from build123d import *

# Parameters (mm, degrees)
SKETCH1_R           = 15
SKETCH1_R_2         = 10
BOSS_EXTRUDE1_DEPTH = 65
SKETCH2_R           = 25
SKETCH2_R_2         = 10
SKETCH2_R_3         = 2.25
BOSS_EXTRUDE2_DEPTH = 4
SKETCH4_R           = 1.4
CUT_EXTRUDE1_DEPTH  = 20
CHAMFER1_SIZE       = 1
CHAMFER2_SIZE       = 0.5
FILLET1_R           = 0.5


with BuildPart() as part:
    # Sketch1 → Boss-Extrude1 (new body)
    with BuildSketch(Plane(origin=(0, 0, 0), x_dir=(1, 0, 0), z_dir=(0, 1, 0))):
        with Locations(Location((0, 0, 0), (0, 0, 270))):
            Circle(SKETCH1_R)
        with Locations(Location((0, 0, 0), (0, 0, 270))):
            Circle(SKETCH1_R_2, mode=Mode.SUBTRACT)
    extrude(amount=BOSS_EXTRUDE1_DEPTH)

    # Sketch2 → Boss-Extrude2 (add)
    with BuildSketch(Plane(origin=(0, 65, 0), x_dir=(1, 0, 0), z_dir=(0, 1, 0))):
        with Locations(Location((0, 0, 0), (0, 0, 270))):
            Circle(SKETCH2_R)
        with Locations(Location((0, 0, 0), (0, 0, 270))):
            Circle(SKETCH2_R_2, mode=Mode.SUBTRACT)
        with Locations(Location((20, 0, 0), (0, 0, 270))):
            Circle(SKETCH2_R_3, mode=Mode.SUBTRACT)
        with Locations(Location((0, -20, 0), (0, 0, 270))):
            Circle(SKETCH2_R_3, mode=Mode.SUBTRACT)
        with Locations(Location((-20, 0, 0), (0, 0, 270))):
            Circle(SKETCH2_R_3, mode=Mode.SUBTRACT)
        with Locations(Location((0, 20, 0), (0, 0, 270))):
            Circle(SKETCH2_R_3, mode=Mode.SUBTRACT)
    extrude(amount=BOSS_EXTRUDE2_DEPTH)

    # Sketch4 → Cut-Extrude1 (cut)
    with BuildSketch(Plane.XZ):
        with Locations(Location((12.5, 0, 0), (0, 0, 270))):
            Circle(SKETCH4_R)
        with Locations(Location((0, -12.5, 0), (0, 0, 270))):
            Circle(SKETCH4_R)
        with Locations(Location((-12.5, 0, 0), (0, 0, 270))):
            Circle(SKETCH4_R)
        with Locations(Location((0, 12.5, 0), (0, 0, 270))):
            Circle(SKETCH4_R)
    extrude(amount=-CUT_EXTRUDE1_DEPTH, mode=Mode.SUBTRACT)

    # Chamfer1
    chamfer1_edges = [part.edges().sort_by_distance(p)[0] for p in [
        (0, 0, -15),
    ]]
    chamfer(chamfer1_edges, length=CHAMFER1_SIZE)

    # Chamfer2
    chamfer2_edges = [part.edges().sort_by_distance(p)[0] for p in [
        (0, 65, -25),
    ]]
    chamfer(chamfer2_edges, length=CHAMFER2_SIZE)

    # Fillet1
    fillet1_edges = [part.edges().sort_by_distance(p)[0] for p in [
        (0, 65, -15),
    ]]
    fillet(fillet1_edges, radius=FILLET1_R)


solid = part.part
Can you work these out from the model? Positions are in its coordinate system, mm. A direction names the side the tool comes from. Coordinates: 2 decimals unless noted, no trailing zeros. Write each loop counter-clockwise with the first axis right and the second up, starting at its lowest first coordinate (ties: lowest second). Pieces come first, ordered by that corner, then holes.
Q1. Please list where these lines run through material, in increasing order: L1, parallel to X at y = 66, z = 20; L2, parallel to X at y = 46, z = 0; L3, parallel to Y at x = 12, z = -14.5.
Results found:
L1: x = -15 to -2.25, 2.25 to 15
L2: x = -15 to -10, 10 to 15
L3: y = 65 to 69
Q2. If we mould it in two halves opening along X, with no side actions, what happens to faces 1 (the face through (13.89, 9.86, 0.18)), 2 (the face through (0.66, 32.306, -14.985)), 3 (the face through (0, 65, 16))? For each: +X half, -X half, draft (parallel to the pull), parting line (faces both ways), or undercut.
Results found:
face 1: undercut
face 2: parting line
face 3: draft
Q3. For P1, Ø12, axis at y = 9.5, z = 15.5, coming from the -X side; P2, Ø8, axis at x = 6, y = 18.5, coming from the +Z side; P3, Ø5, axis at y = 17.5, z = -9, coming from the +X side, each with a flat end and sliding along its axis, tell me the tip position at first contact or that it passes through.
Results found:
P1: stops at x = -11.61
P2: stops at z = 14.87
P3: stops at x = 13.52
Q4. Imagine slicing it at C-C, the plane y = 23. List the corners of the cut face in (x, z) for me.
Results found:
outline: circle Ø30 at (0, 0); hole circle Ø20 at (0, 0)
Q5. Which directions (+Z, -Z, +X, -X, +Y, -Y) give clear straight access to the entire face, cutting with the end or side of a thin tool? Please do faces 4 (the face through (-9.76, 34.02, -2.17)), 5 (the face through (-12, 20, 0)).
Results found:
face 4: +Y, -Y
face 5: -Y
Q6. Imagine slicing it at A-A, the plane z = 0. Count the separate pieces of the cut face and the enclosed holes in it, plus the area to 3 significant figures.
Results found:
separate pieces: 4
enclosed holes: 0
area: 621 mm2
